from build123d import *

# Parameters (mm, degrees)
F0_W     = 55.42358
F0_H     = 46.27962
F1_DEPTH = 40
F2_R     = 6.761924
F2_R_2   = 6.673414
F2_R_3   = 6.092798
F2_R_4   = 6.349814
F3_DEPTH = 5
F4_W     = 51.318126
F4_H     = 42.360786
F4_R     = 6.730957
F5_DEPTH = 25


with BuildPart() as f1:
    # F0 (on Top) → F1 (new body)
    with BuildSketch(Plane.XY):
        with Locations((27.71179, 23.13981)):
            Rectangle(F0_W, F0_H)
    extrude(amount=F1_DEPTH)

    # F2 (on face) → F3 (join)
    with BuildSketch(Plane.XY.offset(40)):
        with Locations((13.249407, 32.656994)):
            Circle(F2_R)
        with Locations((43.293841, 31.910546)):
            Circle(F2_R_2)
        with Locations((14.182466, 10.077015)):
            Circle(F2_R_3)
        with Locations((43.10723, 10.077015)):
            Circle(F2_R_4)
    extrude(amount=F3_DEPTH)

    # F4 (on face) → F5 (cut)
    with BuildSketch(Plane(origin=(0, 0, 0), x_dir=(1, 0, 0), z_dir=(0, 0, -1))):
        with Locations((27.8984, -23.233118)):
            Rectangle(F4_W, F4_H)
        with Locations((28.178319, -23.513034)):
            Circle(F4_R, mode=Mode.SUBTRACT)
    extrude(amount=-F5_DEPTH, mode=Mode.SUBTRACT)


solid = f1.part
Geometry check sheet. Reference: the model listing, model coordinates, mm. A direction names the side the tool comes from. Round coordinates to 2 decimals unless told otherwise and drop trailing zeros. Loops run counter-clockwise (first coordinate to the right, second up) from the corner with the lowest first, then second, coordinate; pieces in that order, holes last. Notation, with made-up numbers: (-9, -17.75) - (33, -17.75) arc R12 cw to (33, -1.75) - close; hole circle Ø9 at (65, 8.5). An arc over 180 degrees is marked (long way). One line per question, with ' | ' between items. Start each with the question number.
1. Cross-section at D-D on x = 28.5. Record the cut outline in (y, z).
2. Scan lines: line 1 (Y direction, x = 8.5, z = 10); line 2 (X direction, y = 7, z = 5); line 3 (X direction, y = 24.5, z = 15.5). Record each from-to range of solid material in increasing order. Write a range as [from, to].
3. Draft check along X on faces 1 (the face through (27, 0, 20)), 2 (the face through (55.424, 23, 20)), 3 (the face through (53.557, 24, 12)). Enter one of: released by +X, released by -X, zero draft, split by the parting line, or undercut.
4. Cross-section at C-C on y = 9. Record the cut outline in (x, z).
5. Depth check by flat-ended pin: pin 1 (8 mm diameter, centred on x = 20.5, y = 10, fed in from -Z); pin 2 (1.5 mm diameter, centred on x = 21.5, y = 24.5, fed in from +Z). Enter the tip coordinate at first touch or a pass-through.
6. Cross-section at A-A on z = 4. Record the cut outline in (x, y).
7. Cross-section at B-B on x = 5.5. Record the cut outline in (y, z), then the cut area to 3 significant figures.
8. Tool access check on faces 4 (the face through (46.037, 4.444, 42.465)), 5 (the face through (2.239, 24, 12)), 6 (the face through (43, 32, 45)). Record the directions out of +Z, -Z, +X, -X, +Y, -Y that give a thin tool (end or side, any length) a straight path to the whole face; none if there is none.
Taken from the geometry:
1) outline: (0, 0) - (2.05, 0) - (2.05, 25) - (16.79, 25) - (16.79, 0) - (30.24, 0) - (30.24, 25) - (44.41, 25) - (44.41, 0) - (46.28, 0) - (46.28, 40) - (0, 40) - close
2) line 1: [0, 2.05], [44.41, 46.28] | line 2: [0, 2.24], [53.56, 55.42] | line 3: [0, 2.24], [21.52, 34.84], [53.56, 55.42]
3) face 1: zero draft | face 2: released by +X | face 3: undercut
4) outline: (0, 0) - (2.24, 0) - (2.24, 25) - (53.56, 25) - (53.56, 0) - (55.42, 0) - (55.42, 40) - (49.37, 40) - (49.37, 45) - (36.85, 45) - (36.85, 40) - (20.18, 40) - (20.18, 45) - (8.19, 45) - (8.19, 40) - (0, 40) - close
5) pin 1: z = 25 | pin 2: z = 40
6) outline: (0, 0) - (55.42, 0) - (55.42, 46.28) - (0, 46.28) - close; circle Ø13.46 at (28.18, 23.51); hole (2.24, 2.05) - (53.56, 2.05) - (53.56, 44.41) - (2.24, 44.41) - close
7) outline: (0, 0) - (2.05, 0) - (2.05, 25) - (44.41, 25) - (44.41, 0) - (46.28, 0) - (46.28, 40) - (0, 40) - close | area: 792 mm²
8) face 4: +Z | face 5: -Z | face 6: +Z, +X, -X, +Y, -Y
